```python
from build123d import *

# Parameters (mm, degrees)
SKETCH1_W           = 25.4
SKETCH1_H           = 139.7
SKETCH1_R           = 3.175
BOSS_EXTRUDE1_DEPTH = 6.35
FILLET2_R           = 12.7
FILLET3_R           = 2.116666667


with BuildPart() as part:
    # Sketch1 → Boss-Extrude1 (new body)
    with BuildSketch(Plane(origin=(0, 0, 0), x_dir=(1, 0, 0), z_dir=(0, 1, 0))):
        Rectangle(SKETCH1_W, SKETCH1_H)
        with Locations(Location((0, -57.15, 0), (0, 0, 270))):
            Circle(SKETCH1_R, mode=Mode.SUBTRACT)
        with Locations(Location((0, 38.1, 0), (0, 0, 270))):
            Circle(SKETCH1_R, mode=Mode.SUBTRACT)
        with Locations(Location((0, 57.15, 0), (0, 0, 270))):
            Circle(SKETCH1_R, mode=Mode.SUBTRACT)
        with Locations(Location((0, -38.1, 0), (0, 0, 270))):
            Circle(SKETCH1_R, mode=Mode.SUBTRACT)
    extrude(amount=BOSS_EXTRUDE1_DEPTH)

    # Fillet2
    fillet2_edges = [part.edges().sort_by_distance(p)[0] for p in [
        (-12.7, 3.175, -69.85),
        (12.7, 3.175, -69.85),
        (-12.7, 3.175, 69.85),
        (12.7, 3.175, 69.85),
    ]]
    fillet(fillet2_edges, radius=FILLET2_R - 0.0001)  # a hair under: the kernel refuses the full size

    # Fillet3
    fillet3_edges = [part.edges().sort_by_distance(p)[0] for p in [
        (-12.7, 0, 0),
        (-12.7, 6.35, 0),
        (12.7, 0, 0),
        (8.98028541, 0, 66.13028541),
        (-8.98028541, 0, 66.13028541),
        (8.98028541, 0, -66.13028541),
        (-8.98028541, 0, -66.13028541),
        (12.7, 6.35, 0),
        (8.98028541, 6.35, 66.13028541),
        (-8.98028541, 6.35, 66.13028541),
        (8.98028541, 6.35, -66.13028541),
        (-8.98028541, 6.35, -66.13028541),
    ]]
    fillet(fillet3_edges, radius=FILLET3_R)


solid = part.part
```
Model file for the job. Use its own axes, mm. Round coordinates to 2 decimals unless told otherwise and drop trailing zeros. Loops run counter-clockwise (first coordinate to the right, second up) from the corner with the lowest first, then second, coordinate; pieces in that order, holes last. Notation, with made-up numbers: M -22,-34.75 L -18,-34.75 A16 ccw -18,-24.75 Z; hole C 64.25,-1.5 d3. An arc over 180 degrees is marked long. Put each result on its own line as item: value. Start each with the question number.
Item 1: Drop flat-ended pins along their axis: P1, Ø5, axis at x = 0, z = 38.1, coming from the +Y side; P2, Ø3, axis at x = 9, y = 3, coming from the +Z side; P3, Ø1.5, axis at x = 5.5, y = 4.5, coming from the +Z side. Give the stop position or say it passes through.
Item 2: Drill centre lines: line 1 along X through (y, z) = (2.25, 38.1) (3 decimals); line 2 along Z through (x, y) = (-2, 3.25); line 3 along Z through (x, y) = (-0.75, 5.5). Where is each one in solid material? Low to high.
Item 3: Cut at D-D (z = 37). List the corners of the cut face in (x, y), then the cut area to 3 significant figures.
Item 4: Mould opens along X. For faces 1 (the face through (8.88, 3.19, -66.23)), 2 (the face through (-9.08, 3.19, 66.03)), 3 (the face through (0.14, 3.13, 53.98)) say: released by +X, released by -X, zero draft, split by the parting line, or undercut.
Item 5: Cut at B-B (y = 1). Give the number of separate pieces and of enclosed holes in the cut face, then the cut area to 3 significant figures.
Item 6: Cut at C-C (z = 2.5). List the corners of the cut face in (x, y), then the cut area to 3 significant figures.
Item 7: Cut at A-A (z = -38.1). List the corners of the cut face in (x, y) (3 decimals).
Answer block:
1. P1: through
1. P2: z = 67.4
1. P3: z = 68.92
2. line 1: -12.7 to -3.175, 3.175 to 12.7
2. line 2: -69.69 to -59.62, -54.68 to -40.57, -35.63 to 35.63, 40.57 to 54.68, 59.62 to 69.69
2. line 3: -69.41 to -60.24, -54.06 to -41.19, -35.01 to 35.01, 41.19 to 54.06, 60.24 to 69.41
3. outline: M -12.7,2.12 A2.12 ccw -10.58,0 L -2.98,0 L -2.98,6.35 L -10.58,6.35 A2.12 ccw -12.7,4.23 Z; M 2.98,0 L 10.58,0 A2.12 ccw 12.7,2.12 L 12.7,4.23 A2.12 ccw 10.58,6.35 L 2.98,6.35 Z
3. area: 120 mm2
4. face 1: released by +X
4. face 2: released by -X
4. face 3: undercut
5. separate pieces: 1
5. enclosed holes: 4
5. area: 3,190 mm2
6. outline: M -12.7,2.12 A2.12 ccw -10.58,0 L 10.58,0 A2.12 ccw 12.7,2.12 L 12.7,4.23 A2.12 ccw 10.58,6.35 L -10.58,6.35 A2.12 ccw -12.7,4.23 Z
6. area: 157 mm2
7. outline: M -12.7,2.117 A2.117 ccw -10.583,0 L -3.175,0 L -3.175,6.35 L -10.583,6.35 A2.117 ccw -12.7,4.233 Z; M 3.175,0 L 10.583,0 A2.117 ccw 12.7,2.117 L 12.7,4.233 A2.117 ccw 10.583,6.35 L 3.175,6.35 Z
